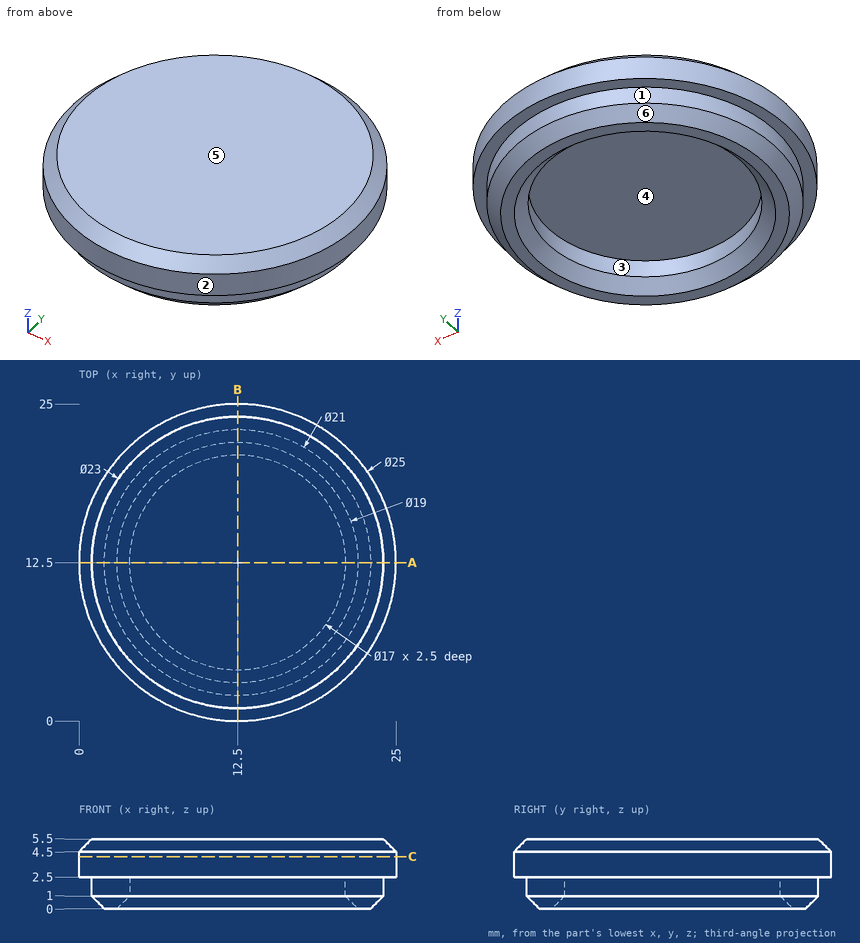
The drawing under review shows one solid part. Ordinate dimensions are in mm from its lowest x, y, z. A direction names the side the tool comes from. Coordinates: 2 decimals unless noted, no trailing zeros. Write each loop counter-clockwise with the first axis right and the second up, starting at its lowest first coordinate (ties: lowest second). Pieces come first, ordered by that corner, then holes. Notation, with made-up numbers: (-15, -34.5) - (21, -34.5) arc R15 cw to (21, -6.5) - close; hole circle Ø3 at (-30, -32). An arc over 180 degrees is marked (long way). Put each result on its own line as item: value.
1. Add section A-A, the plane y = 12.5. Give the boundary of the cut face in (x, z), then the cut area to 3 significant figures.
Values found:
outline: (0, 2.5) - (1, 2.5) - (1, 1) - (2, 0) - (3, 0) - (4, 1) - (4, 2.5) - (21, 2.5) - (21, 1) - (22, 0) - (23, 0) - (24, 1) - (24, 2.5) - (25, 2.5) - (25, 4.5) - (24, 5.5) - (1, 5.5) - (0, 4.5) - close
area: 87.0 mm²
2. Add section C-C, the plane z = 4.1. Give the boundary of the cut face in (x, y).
Values found:
outline: circle Ø25 at (12.5, 12.5)
3. Mouldability with a two-part tool opening along Y and no side actions: class the marked faces 3, 4, 5 and 6 as released by +Y, released by -Y, zero draft, split by the parting line, or undercut.
Values found:
face 3: undercut
face 4: undercut
face 5: zero draft
face 6: split by the parting line
4. Wall thickness on probe 1 along Y at (x, z) = (12.5, 2.05); probe 2 along Z at (x, y) = (20.5, 13); probe 3 along X at (y, z) = (6, 4): over which ranges is each line inside the solid? List them lowest first.
Values found:
probe 1: 1 to 4, 21 to 24
probe 2: 2.5 to 5.5
probe 3: 1.82 to 23.18
5. Machinability: for the marked faces 1 and 2, which of the approach directions +Z, -Z, +X, -X, +Y, -Y give a long, thin tool a straight path to every point of the face, cutting with its end or side? Answer none if there is none.
Values found:
face 1: -Z
face 2: +Z, -Z
6. For pin 1 (1.5 mm diameter, centred on y = 18.5, z = 3, fed in from -X), flat-tipped, find the tip position at first contact; note if it passes through.
Values found:
pin 1: x = 1.16
